```python
from build123d import *

# Parameters (mm, degrees)
SKETCH1_W                  = 6.5
SKETCH1_H                  = 12.5
MAIN_BASE_DEPTH            = 11
TOP_LINK_HOLES_DEPTH       = 16.1
STEERING_MOUNT_BOSS_DEPTH  = 4
CUT_FOR_LINK_DEPTH         = 4.1
BOSS_EXTRUDE6_REACH        = 28.238
SKETCH4_R                  = 2.5
STEERING_MOUNT_HOLES_DEPTH = 41.847064
SKETCH13_R                 = 1.5
CUT_EXTRUDE8_DEPTH         = 15
CUT_EXTRUDE9_REACH         = 13.5
SKETCH14_R                 = 4.75
SKETCH15_R                 = 1.5
CUT_EXTRUDE10_DEPTH        = 16.1


with BuildPart() as part:
    # Sketch1 → Main Base (new body)
    with BuildSketch(Plane.XY):
        with BuildLine():
            Line((0, 0), (-10.5, 0))
            Line((-10.5, 0), (-10.693077779, 1.572492321))
            Line((-10.693077779, 1.572492321), (-23.5, 0))
            Line((-23.5, 0), (-23.5, 6.045058953))
            Line((-23.5, 6.045058953), (-11.42429384, 7.527769231))
            Line((-11.42429384, 7.527769231), (-12.359894337, 15.1476238))
            ThreePointArc((-12.359894337, 15.1476238), (-9.125383898, 21.988425282), (-11.433037505, 29.194905528))
            Line((-11.433037505, 29.194905528), (-16.182087698, 34.999776092))
            Line((-16.182087698, 34.999776092), (-16.669565072, 38.969960698))
            Line((-16.669565072, 38.969960698), (-21.343327687, 38.396094808))
            Line((-21.343327687, 38.396094808), (-21.83080506, 42.366279414))
            Line((-21.83080506, 42.366279414), (-16.669565072, 43))
            Line((-16.669565072, 43), (-0.569565072, 43))
            Line((-0.569565072, 43), (-0.569565072, 34.310888907))
            ThreePointArc((-0.569565072, 34.310888907), (2.730584507, 23.23242246), (0, 12))
            Line((0, 12), (0, 0))
        make_face()
        with Locations((-5.25, 8.25)):
            Rectangle(SKETCH1_W, SKETCH1_H, mode=Mode.SUBTRACT)
    extrude(amount=MAIN_BASE_DEPTH)

    # Sketch2 → Top Link Holes (add)
    with BuildSketch(Plane(origin=(-0.569565072, 0, 0), x_dir=(0, 0, -1), z_dir=(1, 0, 0))):
        with BuildLine():
            Line((-11, 43), (-11, 45))
            ThreePointArc((-11, 45), (-6.75, 49.25), (-2.5, 45))
            Line((-2.5, 45), (-2.5, 43))
            Line((-2.5, 43), (-11, 43))
        make_face()
    extrude(amount=-TOP_LINK_HOLES_DEPTH)

    # Sketch3 → Steering Mount Boss (add)
    with BuildSketch(Plane(origin=(-5.448899417, 44.377724505, 0), x_dir=(0.992546152, 0.121869343, 0), z_dir=(-0.121869343, 0.992546152, 0))):
        with BuildLine():
            Line((-16.504930895, 0), (-16.504930895, -11))
            ThreePointArc((-16.504930895, -11), (-22.004930895, -5.5), (-16.504930895, 0))
        make_face()
    extrude(amount=-STEERING_MOUNT_BOSS_DEPTH)

    # Sketch5 → Cut for Link (cut, symmetric)
    with BuildSketch(Plane(origin=(-7.819565072, 0, 0), x_dir=(0, 0, -1), z_dir=(1, 0, 0))):
        with BuildLine():
            Line((-11, 32.5), (0, 35))
            Line((0, 35), (0, 43))
            Line((0, 43), (-2.5, 43))
            Line((-2.5, 43), (-2.5, 45))
            ThreePointArc((-2.5, 45), (-6.75, 49.25), (-11, 45))
            Line((-11, 45), (-11, 32.5))
        make_face()
    extrude(amount=CUT_FOR_LINK_DEPTH, both=True, mode=Mode.SUBTRACT)

    # Boss-Extrude6: up to this face of the body (flat: up to its plane)
    boss_extrude6_end = Plane(part.part.faces().sort_by_distance((-11.892094088, 11.337696516, 5.5))[0])
    # Sketch12 → Boss-Extrude6 (add, up to the picked face)
    with BuildSketch(Plane.ZY.offset(23.5), mode=Mode.PRIVATE) as boss_extrude6_sk1:
        with BuildLine():
            Line((11, 6.045058953), (0, 6.045058953))
            Line((0, 6.045058953), (0, 4.853970757))
            ThreePointArc((0, 4.853970757), (-1.35322413, 6.175171241), (-1.85, 8))
            Line((-1.85, 8), (-1.85, 11.5))
            Line((-1.85, 11.5), (5.65, 11.5))
            Line((5.65, 11.5), (11, 6.045058953))
        make_face()
    boss_extrude6_tool1 = split(extrude(boss_extrude6_sk1.sketch, amount=-BOSS_EXTRUDE6_REACH, mode=Mode.PRIVATE), bisect_by=boss_extrude6_end, keep=Keep.BOTH, mode=Mode.PRIVATE)
    add(boss_extrude6_tool1.solids().sort_by_distance((-23.5, 8.500537, 3.327239))[0])

    # Sketch4 → Steering mount holes (cut)
    with BuildSketch(Plane(origin=(-5.448899417, 44.377724505, 0), x_dir=(0.992546152, 0.121869343, 0), z_dir=(-0.121869343, 0.992546152, 0))):
        with Locations((-16.504930895, -5.5)):
            Circle(SKETCH4_R)
    extrude(amount=-STEERING_MOUNT_HOLES_DEPTH, mode=Mode.SUBTRACT)

    # Sketch13 → Cut-Extrude8 (cut)
    with BuildSketch(Plane.ZY.offset(23.5)):
        with Locations((1.75, 8)):
            Circle(SKETCH13_R)
    extrude(amount=-CUT_EXTRUDE8_DEPTH, mode=Mode.SUBTRACT)

    # Cut-Extrude9: up to this face of the body (flat: up to its plane)
    cut_extrude9_end = Plane(part.part.faces().sort_by_distance((-15.449529226, 7.033532472, 10.515271267))[0])
    # Sketch14 → Cut-Extrude9 (cut, up to the picked face)
    with BuildSketch(Plane(origin=(0, 11.5, 0), x_dir=(1, 0, 0), z_dir=(0, 1, 0)), mode=Mode.PRIVATE) as cut_extrude9_sk1:
        with Locations((-18.040902496, -5.5)):
            Circle(SKETCH14_R)
    cut_extrude9_tool1 = split(extrude(cut_extrude9_sk1.sketch, amount=-CUT_EXTRUDE9_REACH, mode=Mode.PRIVATE), bisect_by=cut_extrude9_end, keep=Keep.BOTH, mode=Mode.PRIVATE)
    add(cut_extrude9_tool1.solids().sort_by_distance((-18.040902, 11.5, 5.5))[0], mode=Mode.SUBTRACT)

    # Sketch15 → Cut-Extrude10 (cut)
    with BuildSketch(Plane(origin=(-0.569565072, 0, 0), x_dir=(0, 0, -1), z_dir=(1, 0, 0))):
        with Locations((-8.25, 45)):
            Circle(SKETCH15_R)
    extrude(amount=-CUT_EXTRUDE10_DEPTH, mode=Mode.SUBTRACT)


solid = part.part
```
Model file for the job. Use its own axes, mm. A direction names the side the tool comes from. Coordinates: 2 decimals unless noted, no trailing zeros. Write each loop counter-clockwise with the first axis right and the second up, starting at its lowest first coordinate (ties: lowest second). Pieces come first, ordered by that corner, then holes. Notation, with made-up numbers: (-18, 59.25) - (3, 59.25) arc R21 cw to (3, 86.25) - close; hole circle Ø4 at (81.5, -35.75). An arc over 180 degrees is marked (long way). One line per item, written item: value. Start each with the question number.
1. Flat gauge pins, fed straight in: pin 1 (3.5 mm diameter, centred on y = 8, z = 1.75, fed in from +X); pin 2 (1 mm diameter, centred on x = -22.5, z = 0, fed in from -Y); pin 3 (6 mm diameter, centred on x = -10, z = 0, fed in from +Y); pin 4 (12 mm diameter, centred on x = -5.5, y = 44, fed in from +Z). Where does each tip first touch, or does it go through?
2. Slice it at C-C (y = 11). Write the cut outline in (x, z).
3. Mould opens along Z. For faces 1 (the cylindrical face through (2.726, 23.396, 5.423)), 2 (the cylindrical face through (-18.66, 9.43, 0.79)), 3 (the cylindrical face through (-14.26, 49.25, 6.84)), 4 (the flat face through (-14, 44, 2.5)) say: released by +Z, released by -Z, zero draft, split by the parting line, or undercut.
4. Slice it at D-D (y = 17). Write the cut outline in (x, z), plus the area to 3 significant figures.
5. Slice it at B-B (y = 44.5). Write the cut outline in (x, z).
6. Tool access for faces 5 (the flat face through (-5, 2, 5)), 6 (the flat face through (-14.9, 7.1, 10.6)), 7 (the flat face through (-23.5, 6, 5)): list every direction of +Z, -Z, +X, -X, +Y, -Y with a clear straight run to the whole face (end or side of a thin tool).
7. Slice it at A-A (x = -7.5). Write the cut outline in (y, z).
8. Probe line 1 (X direction, y = 7.5, z = 5.5); line 2 (X direction, y = 45, z = 3.25); line 3 (X direction, y = 38.5, z = 6). List the from-to ranges inside material, lowest first. Write a range as from..to.
Answers below:
1. pin 1: stops at x = 0
1. pin 2: stops at y = 0.06
1. pin 3: stops at y = 43
1. pin 4: stops at z = 11
2. outline: (-23.5, -1.85) - (-11.85, -1.85) - (-11.85, 0) - (-8.5, 0) - (-8.5, 11) - (-11.85, 11) - (-11.85, 6.14) - (-13.33, 6.14) arc R4.75 cw (long way) to (-22.75, 6.14) - (-23.5, 6.14) - close; (-2, 0) - (0, 0) - (0, 11) - (-2, 11) - close
3. face 1: zero draft
3. face 2: undercut
3. face 3: split by the parting line
3. face 4: released by -Z
4. outline: (-10.8, 0) - (2, 0) - (2, 11) - (-10.8, 11) - close
4. area: 141 mm^2
5. outline: (-16.67, 2.5) - (-11.92, 2.5) - (-11.92, 6.84) - (-16.67, 6.84) - close; (-16.67, 9.66) - (-11.92, 9.66) - (-11.92, 11) - (-16.67, 11) - close; (-3.72, 2.5) - (-0.57, 2.5) - (-0.57, 6.84) - (-3.72, 6.84) - close; (-3.72, 9.66) - (-0.57, 9.66) - (-0.57, 11) - (-3.72, 11) - close
6. face 5: +Z, -Z
6. face 6: +Z, -X
6. face 7: +Z, -Z, -X, -Y
7. outline: (0, 0) - (2, 0) - (2, 11) - (0, 11) - close; (14.5, 0) - (35, 0) - (32.5, 11) - (14.5, 11) - close
8. line 1: x = -23.5..-22.79, -13.29..-8.5, -2..0
8. line 2: x = -16.67..-11.92, -3.72..-0.57
8. line 3: x = -26.87..-23.82, -16.61..-11.92, -3.72..-0.57
